The model under review builds one solid part; all positions refer to its coordinate system, in mm. A direction names the side the tool comes from. Coordinates: 2 decimals unless noted, no trailing zeros. Loops run counter-clockwise (first coordinate to the right, second up) from the corner with the lowest first, then second, coordinate; pieces in that order, holes last. Notation, with made-up numbers: (-20, 84.5) - (-9, 84.5) arc R19 cw to (-9, 108.5) - close; hole circle Ø7 at (43, -36). An arc over 180 degrees is marked (long way). Answer in a Markdown table with one row per item. Add a question column.
(1) For line 1 along Y through (x, z) = (20, 3.9); line 2 along Y through (x, z) = (36, 1.15); line 3 along Y through (x, z) = (30, 3.7), list the stretches that pass through material, from the lowest coordinate up.
(2) We need section A-A on x = 180. Write out the cut boundary in (y, z), plus the area to 3 significant figures.
(3) We need section B-B on z = 2.45. Give the number of separate pieces and of enclosed holes in the cut face, plus the area to 3 significant figures.
(4) Machinability: for faces 1 (the flat face through (157, 73, 0)), 2 (the flat face through (50.21, 204.18, 2.46)), which of the approach directions +Z, -Z, +X, -X, +Y, -Y give a long, thin tool a straight path to every point of the face, cutting with its end or side? Answer none if there is none.
(5) We need section C-C on x = 249. Write out the cut boundary in (y, z).
(6) For P1, Ø1.5, axis at x = 57.5, z = 1.5, coming from the +Y side; P2, Ø1.5, axis at y = 253.5, z = 3, coming from the -X side; P3, Ø2.5, axis at y = 115, z = 1.5, coming from the +X side, all flat-tipped, find the tip position at first contact; note any pin that passes through.
(7) Mouldability with a two-part tool opening along X and no side actions: class faces 3 (the flat face through (20, 235, 2)), 4 (the flat face through (260.21, 203.76, 2.46)), 5 (the flat face through (157, 73, 5)) as +X half, -X half, draft (parallel to the pull), parting line (faces both ways), or undercut.
from build123d import *

# Parameters (mm, degrees)
SKIZZE1_R                       = 1.6
AUFSATZ_LINEAR_AUSTRAGEN1_DEPTH = 5


with BuildPart() as part:
    # Skizze1 → Aufsatz-Linear austragen1 (new body)
    with BuildSketch(Plane.XY):
        Polygon((5, 10), (5, 20), (0, 20), (0, 30), (5, 30), (5, 40), (0, 40), (0, 50), (5, 50), (5, 60), (0, 60), (0, 70), (5, 70), (5, 80), (0, 80), (0, 90), (5, 90), (5, 100), (0, 100), (0, 110), (5, 110), (5, 120), (0, 120), (0, 130), (5, 130), (5, 140), (0, 140), (0, 150), (5, 150), (5, 160), (0, 160), (0, 170), (5, 170), (5, 180), (0, 180), (0, 190), (5, 190), (5, 200), (0, 200), (0, 210), (5, 210), (5, 220), (35, 250), (45, 250), (45, 255), (55, 255), (55, 250), (65, 250), (65, 255), (75, 255), (75, 250), (85, 250), (85, 255), (95, 255), (95, 250), (105, 250), (105, 255), (115, 255), (115, 250), (125, 250), (125, 255), (135, 255), (135, 250), (145, 250), (145, 255), (155, 255), (155, 250), (165, 250), (165, 255), (175, 255), (175, 250), (185, 250), (185, 255), (195, 255), (195, 250), (205, 250), (205, 255), (215, 255), (215, 250), (225, 250), (225, 255), (235, 255), (235, 250), (245, 250), (245, 255), (255, 255), (255, 250), (265, 250), (265, 255), (275, 255), (275, 250), (305, 220), (305, 210), (310, 210), (310, 200), (305, 200), (305, 190), (310, 190), (310, 180), (305, 180), (305, 170), (310, 170), (310, 160), (305, 160), (305, 150), (310, 150), (310, 140), (305, 140), (305, 130), (310, 130), (310, 120), (305, 120), (305, 110), (310, 110), (310, 100), (305, 100), (305, 90), (310, 90), (310, 80), (305, 80), (305, 70), (310, 70), (310, 60), (305, 60), (305, 50), (310, 50), (310, 40), (305, 40), (305, 30), (310, 30), (310, 20), (305, 20), (305, 10), (310, 10), (310, 0), (305, 0), (5, 0), (0, 0), (0, 10), align=None)
        with Locations((290, 214.999999999)):
            Circle(SKIZZE1_R, mode=Mode.SUBTRACT)
        with Locations((280, 214.999999999)):
            Circle(SKIZZE1_R, mode=Mode.SUBTRACT)
        with Locations((20, 215)):
            Circle(SKIZZE1_R, mode=Mode.SUBTRACT)
        with Locations((30, 215)):
            Circle(SKIZZE1_R, mode=Mode.SUBTRACT)
        with Locations((20, 36)):
            Circle(SKIZZE1_R, mode=Mode.SUBTRACT)
        with Locations((155, 36)):
            Circle(SKIZZE1_R, mode=Mode.SUBTRACT)
        with Locations((290, 36)):
            Circle(SKIZZE1_R, mode=Mode.SUBTRACT)
        Polygon((275, 188.971165398), (245, 218.971165398), (65, 218.971165398), (35, 188.971165398), (35, 78.971165398), (275, 78.971165398), align=None, mode=Mode.SUBTRACT)
    extrude(amount=AUFSATZ_LINEAR_AUSTRAGEN1_DEPTH)


solid = part.part
Outcome:
| question | item | result |
|---|---|---|
| 1 | line 1 | 0 to 34.4, 37.6 to 213.4, 216.6 to 235 |
| 1 | line 2 | 0 to 78.97, 189.97 to 250 |
| 1 | line 3 | 0 to 213.4, 216.6 to 245 |
| 2 | outline | (0, 0) - (78.97, 0) - (78.97, 5) - (0, 5) - close; (218.97, 0) - (250, 0) - (250, 5) - (218.97, 5) - close |
| 2 | area | 550 mm² |
| 3 | separate pieces | 1 |
| 3 | enclosed holes | 8 |
| 3 | area | 43,000 mm² |
| 4 | face 1 | -Z, +X, -X, +Y, -Y |
| 4 | face 2 | +Z, -Z |
| 5 | outline | (0, 0) - (78.97, 0) - (78.97, 5) - (0, 5) - close; (214.97, 0) - (255, 0) - (255, 5) - (214.97, 5) - close |
| 6 | P1 | y = 250 |
| 6 | P2 | x = 45 |
| 6 | P3 | x = 305 |
| 7 | face 3 | -X half |
| 7 | face 4 | undercut |
| 7 | face 5 | draft |
